Build history of the part. All positions in model axes, mm. A direction names the side the tool comes from. Give positions to 0.01 mm unless a question says otherwise; leave off trailing zeros. Order: outer loops, then holes, each group sorted by start corner. A loop starts at its lowest first (then second) coordinate and runs counter-clockwise, first axis right, second up. Notation, with made-up numbers: (-36, 13.5) - (-23, 13.5) arc R16 ccw to (-23, 41.5) - close; hole circle Ø9 at (19, 47.5). An arc over 180 degrees is marked (long way). Answer in a Markdown table with one row per item.
```python
from build123d import *

# Parameters (mm, degrees)
EXTRUDE_1_DEPTH     = 7
SKETCH_2_R          = 6
CUT_EXTRUDE_1_DEPTH = 5
CUT_EXTRUDE_2_DEPTH = 0.5
FILLET_1_R          = 1
SKETCH_4_R          = 1.5
EXTRUDE_3_DEPTH     = 2.5
SKETCH_5_W          = 1.5
SKETCH_5_H          = 4.3
CUT_EXTRUDE_3_DEPTH = 2.5
SKETCH_6_W          = 3.174285876
SKETCH_6_H          = 3
CUT_EXTRUDE_4_DEPTH = 1


with BuildPart() as part:
    # Эскиз1 → Бобышка-Вытянуть1 (new body)
    with BuildSketch(Plane.XY):
        with BuildLine():
            Line((1.201755047, 83), (6.798244953, 83))
            ThreePointArc((6.798244953, 83), (7.648014096, 82.648014096), (8, 81.798244953))
            Line((8, 81.798244953), (8, 32.201755047))
            ThreePointArc((8, 32.201755047), (7.648014096, 31.351985904), (6.798244953, 31))
            Line((6.798244953, 31), (1.201755047, 31))
            ThreePointArc((1.201755047, 31), (0.351985904, 30.648014096), (0, 29.798244953))
            Line((0, 29.798244953), (0, 1.201755047))
            ThreePointArc((0, 1.201755047), (0.351985904, 0.351985904), (1.201755047, 0))
            Line((1.201755047, 0), (163.798244953, 0))
            ThreePointArc((163.798244953, 0), (164.648014096, 0.351985904), (165, 1.201755047))
            Line((165, 1.201755047), (165, 29.798244953))
            ThreePointArc((165, 29.798244953), (164.648014096, 30.648014096), (163.798244953, 31))
            Line((163.798244953, 31), (158.201755047, 31))
            ThreePointArc((158.201755047, 31), (157.351985904, 31.351985904), (157, 32.201755047))
            Line((157, 32.201755047), (157, 81.798244953))
            ThreePointArc((157, 81.798244953), (157.351985904, 82.648014096), (158.201755047, 83))
            Line((158.201755047, 83), (163.798244953, 83))
            ThreePointArc((163.798244953, 83), (164.648014096, 83.351985904), (165, 84.201755047))
            Line((165, 84.201755047), (165, 111.798244953))
            ThreePointArc((165, 111.798244953), (164.648014096, 112.648014096), (163.798244953, 113))
            Line((163.798244953, 113), (1.201755047, 113))
            ThreePointArc((1.201755047, 113), (0.351985904, 112.648014096), (0, 111.798244953))
            Line((0, 111.798244953), (0, 84.201755047))
            ThreePointArc((0, 84.201755047), (0.351985904, 83.351985904), (1.201755047, 83))
        make_face()
    extrude(amount=EXTRUDE_1_DEPTH)

    # Эскиз2 → Вырез-Вытянуть1 (cut)
    with BuildSketch(Plane(origin=(0, 0, 0), x_dir=(-1, 0, 0), z_dir=(0, 0, -1))):
        with BuildLine():
            Line((-161.798244953, 111), (-3.201755047, 111))
            ThreePointArc((-3.201755047, 111), (-2.351985904, 110.648014096), (-2, 109.798244953))
            Line((-2, 109.798244953), (-2, 86.201755047))
            ThreePointArc((-2, 86.201755047), (-2.351985904, 85.351985904), (-3.201755047, 85))
            Line((-3.201755047, 85), (-8.798244953, 85))
            ThreePointArc((-8.798244953, 85), (-9.648014096, 84.648014096), (-10, 83.798244953))
            Line((-10, 83.798244953), (-10, 30.201755047))
            ThreePointArc((-10, 30.201755047), (-9.648014096, 29.351985904), (-8.798244953, 29))
            Line((-8.798244953, 29), (-3.201755047, 29))
            ThreePointArc((-3.201755047, 29), (-2.351985904, 28.648014096), (-2, 27.798244953))
            Line((-2, 27.798244953), (-2, 3.201755047))
            ThreePointArc((-2, 3.201755047), (-2.351985904, 2.351985904), (-3.201755047, 2))
            Line((-3.201755047, 2), (-161.798244953, 2))
            ThreePointArc((-161.798244953, 2), (-162.648014096, 2.351985904), (-163, 3.201755047))
            Line((-163, 3.201755047), (-163, 27.798244953))
            ThreePointArc((-163, 27.798244953), (-162.648014096, 28.648014096), (-161.798244953, 29))
            Line((-161.798244953, 29), (-156.201755047, 29))
            ThreePointArc((-156.201755047, 29), (-155.351985904, 29.351985904), (-155, 30.201755047))
            Line((-155, 30.201755047), (-155, 70.5))
            Line((-155, 70.5), (-155, 74.8))
            Line((-155, 74.8), (-155, 83.798244953))
            ThreePointArc((-155, 83.798244953), (-155.351985904, 84.648014096), (-156.201755047, 85))
            Line((-156.201755047, 85), (-161.798244953, 85))
            ThreePointArc((-161.798244953, 85), (-162.648014096, 85.351985904), (-163, 86.201755047))
            Line((-163, 86.201755047), (-163, 109.798244953))
            ThreePointArc((-163, 109.798244953), (-162.648014096, 110.648014096), (-161.798244953, 111))
        make_face()
        with Locations((-82.5, 57)):
            Circle(SKETCH_2_R, mode=Mode.SUBTRACT)
    extrude(amount=-CUT_EXTRUDE_1_DEPTH, mode=Mode.SUBTRACT)

    # Эскиз3 → Вырез-Вытянуть2 (cut)
    # profile 1 of 2: a face of its own
    with BuildSketch(Plane(origin=(0, 0, 5), x_dir=(-1, 0, 0), z_dir=(0, 0, -1))):
        with BuildLine():
            Line((-120, 31), (-103, 31))
            ThreePointArc((-103, 31), (-102.292893219, 30.707106781), (-102, 30))
            Line((-102, 30), (-102, 19))
            ThreePointArc((-102, 19), (-102.292893219, 18.292893219), (-103, 18))
            Line((-103, 18), (-120, 18))
            ThreePointArc((-120, 18), (-120.707106781, 18.292893219), (-121, 19))
            Line((-121, 19), (-121, 30))
            ThreePointArc((-121, 30), (-120.707106781, 30.707106781), (-120, 31))
        make_face()
    # profile 2 of 2: a face of its own
    with BuildSketch(Plane(origin=(0, 0, 5), x_dir=(-1, 0, 0), z_dir=(0, 0, -1))):
        with BuildLine():
            Line((-52.1501229, 97.239252875), (-39.1501229, 97.239252875))
            ThreePointArc((-39.1501229, 97.239252875), (-38.443016119, 96.946359657), (-38.1501229, 96.239252875))
            Line((-38.1501229, 96.239252875), (-38.1501229, 83.239252875))
            ThreePointArc((-38.1501229, 83.239252875), (-38.443016119, 82.532146094), (-39.1501229, 82.239252875))
            Line((-39.1501229, 82.239252875), (-52.1501229, 82.239252875))
            ThreePointArc((-52.1501229, 82.239252875), (-52.857229681, 82.532146094), (-53.1501229, 83.239252875))
            Line((-53.1501229, 83.239252875), (-53.1501229, 96.239252875))
            ThreePointArc((-53.1501229, 96.239252875), (-52.857229681, 96.946359657), (-52.1501229, 97.239252875))
        make_face()
        Polygon((-41.403231286, 94.64375803), (-44.490035641, 94.64375803), (-48.784719961, 93.637191392), (-48.784719961, 92.630624755), (-44.490035641, 93.637191392), (-41.403231286, 93.637191392), align=None, mode=Mode.SUBTRACT)
        Polygon((-48.784719961, 91.774831443), (-44.490035641, 92.630624755), (-44.490035641, 91.774831443), (-48.784719961, 90.91903813), align=None, mode=Mode.SUBTRACT)
        Polygon((-48.784719961, 90.055112789), (-44.490035641, 90.910906102), (-44.490035641, 90.055112789), (-48.784719961, 89.067866896), align=None, mode=Mode.SUBTRACT)
        Polygon((-48.784719961, 88.216527408), (-44.490035641, 89.067866896), (-41.403231286, 89.067866896), (-41.403231286, 88.316883581), (-44.341167482, 88.316883581), (-48.784719961, 87.436033812), align=None, mode=Mode.SUBTRACT)
        Polygon((-48.609605566, 93.888102843), (-44.858812452, 94.806018458), (-44.858812452, 95.913847648), (-46.734209009, 95.170019477), (-48.609605566, 95.739760204), align=None, mode=Mode.SUBTRACT)
        Polygon((-48.609605566, 87.006809767), (-44.858812452, 87.715709289), (-44.858812452, 86.328076183), (-46.734209009, 86.674984459), (-48.609605566, 85.770006347), align=None, mode=Mode.SUBTRACT)
    extrude(amount=-CUT_EXTRUDE_2_DEPTH, mode=Mode.SUBTRACT)

    # Скругление1
    fillet_1_edges = [part.edges().sort_by_distance(p)[0] for p in [
        (155, 57, 5),
        (155.351985904, 84.648014096, 5),
        (159, 85, 5),
        (162.648014096, 85.351985904, 5),
        (163, 98, 5),
        (162.648014096, 110.648014096, 5),
        (82.5, 111, 5),
        (2.351985904, 110.648014096, 5),
        (2, 98, 5),
        (2.351985904, 85.351985904, 5),
        (6, 85, 5),
        (9.648014096, 84.648014096, 5),
        (10, 57, 5),
        (9.648014096, 29.351985904, 5),
        (6, 29, 5),
        (2.351985904, 28.648014096, 5),
        (2, 15.5, 5),
        (2.351985904, 2.351985904, 5),
        (82.5, 2, 5),
        (162.648014096, 2.351985904, 5),
        (163, 15.5, 5),
        (162.648014096, 28.648014096, 5),
        (159, 29, 5),
        (155.351985904, 29.351985904, 5),
    ]]
    fillet(fillet_1_edges, radius=FILLET_1_R)

    # Эскиз4 → Бобышка-Вытянуть3 (add)
    # profile 1 of 2: a face of its own
    with BuildSketch(Plane(origin=(0, 0, 0), x_dir=(-1, 0, 0), z_dir=(0, 0, -1))):
        with BuildLine():
            Line((-157, 73), (-163.5, 73))
            ThreePointArc((-163.5, 73), (-164.207106781, 72.707106781), (-164.5, 72))
            Line((-164.5, 72), (-164.5, 41))
            ThreePointArc((-164.5, 41), (-164.207106781, 40.292893219), (-163.5, 40))
            Line((-163.5, 40), (-157, 40))
            Line((-157, 40), (-157, 73))
        make_face()
        with Locations((-161.7, 47)):
            Circle(SKETCH_4_R, mode=Mode.SUBTRACT)
        with Locations((-161.7, 65)):
            Circle(SKETCH_4_R, mode=Mode.SUBTRACT)
    # profile 2 of 2: a face of its own
    with BuildSketch(Plane(origin=(0, 0, 0), x_dir=(-1, 0, 0), z_dir=(0, 0, -1))):
        with BuildLine():
            Line((-1.5, 73), (-8, 73))
            Line((-8, 73), (-8, 40))
            Line((-8, 40), (-1.5, 40))
            ThreePointArc((-1.5, 40), (-0.792893219, 40.292893219), (-0.5, 41))
            Line((-0.5, 41), (-0.5, 72))
            ThreePointArc((-0.5, 72), (-0.792893219, 72.707106781), (-1.5, 73))
        make_face()
        with Locations((-3.3, 47)):
            Circle(SKETCH_4_R, mode=Mode.SUBTRACT)
        with Locations((-3.3, 65)):
            Circle(SKETCH_4_R, mode=Mode.SUBTRACT)
    extrude(amount=-EXTRUDE_3_DEPTH)

    # Эскиз5 → Вырез-Вытянуть3 (cut)
    with BuildSketch(Plane(origin=(0, 0, 0), x_dir=(-1, 0, 0), z_dir=(0, 0, -1))):
        with Locations((-155.75, 72.65)):
            Rectangle(SKETCH_5_W, SKETCH_5_H)
    extrude(amount=-CUT_EXTRUDE_3_DEPTH, mode=Mode.SUBTRACT)

    # Эскиз6 → Вырез-Вытянуть4 (cut)
    with BuildSketch(Plane(origin=(0, 0, 0), x_dir=(-1, 0, 0), z_dir=(0, 0, -1))):
        with Locations((-156.587142938, 81.5)):
            Rectangle(SKETCH_6_W, SKETCH_6_H)
    extrude(amount=-CUT_EXTRUDE_4_DEPTH, mode=Mode.SUBTRACT)


solid = part.part
```
1. Cut at C-C on x = 23.5. Write the cut outline in (y, z).
Check result:
| item | result |
|---|---|
| outline | (0, 0) - (2, 0) - (2, 4) arc R1 cw to (3, 5) - (110, 5) arc R1 cw to (111, 4) - (111, 0) - (113, 0) - (113, 7) - (0, 7) - close |
2. Cut at D-D on y = 25.5. Write the cut outline in (x, z).
Check result:
| item | result |
|---|---|
| outline | (0, 0) - (2, 0) - (2, 4) arc R1 cw to (3, 5) - (102, 5) - (102, 5.5) - (121, 5.5) - (121, 5) - (162, 5) arc R1 cw to (163, 4) - (163, 0) - (165, 0) - (165, 7) - (0, 7) - close |
3. Cut at B-B on y = 99.5. Write the cut outline in (x, z), and give its area (3 significant figures).
Check result:
| item | result |
|---|---|
| outline | (0, 0) - (2, 0) - (2, 4) arc R1 cw to (3, 5) - (162, 5) arc R1 cw to (163, 4) - (163, 0) - (165, 0) - (165, 7) - (0, 7) - close |
| area | 350 mm² |
4. Drop flat-ended pins along their axis: P1, Ø1.5, axis at x = 52, y = 25.5, coming from the -Z side; P2, Ø6, axis at x = 3, y = 54.5, coming from the +Z side; P3, Ø1.2, axis at y = 49.5, z = 1, coming from the +X side. Give the stop position or say it passes through.
Check result:
| item | result |
|---|---|
| P1 | stops at z = 5 |
| P2 | stops at z = 2.5 |
| P3 | stops at x = 164.5 |
5. Cut at A-A on x = 82.5. Write the cut outline in (y, z), and give its area (3 significant figures).
Check result:
| item | result |
|---|---|
| outline | (0, 0) - (2, 0) - (2, 4) arc R1 cw to (3, 5) - (51, 5) - (51, 0) - (63, 0) - (63, 5) - (110, 5) arc R1 cw to (111, 4) - (111, 0) - (113, 0) - (113, 7) - (0, 7) - close |
| area | 306 mm² |
6. Which spindle directions (+Z, -Z, +X, -X, +Y, -Y) get a long thin tool onto all of the face, cutting with end or side? Do faces 4 (the face through (4, 57, 2.5)), 5 (the face through (161, 57, 2.5)), 6 (the face through (2, 98, 2)). Say none if no direction does.
Check result:
| item | result |
|---|---|
| face 4 | +Z, -X |
| face 5 | +Z, +X |
| face 6 | -Z |
7. Probe line 1 (X direction, y = 65, z = 0.9); line 2 (Y direction, x = 8.5, z = 2); line 3 (X direction, y = 53, z = 2.75). List the from-to ranges inside material, lowest first.
Check result:
| item | result |
|---|---|
| line 1 | x = 0.5 to 1.8, 4.8 to 10, 155 to 160.2, 163.2 to 164.5 |
| line 2 | y = 0 to 2, 29 to 85, 111 to 113 |
| line 3 | x = 8 to 10, 78.03 to 86.97, 155 to 157 |
8. Two-plate mould, pull along Y, no slides. Class faces 1 (the face through (0, 16, 3)), 2 (the face through (157, 57, 4)), 3 (the face through (81, 0, 3)): +Y half, -Y half, draft (parallel to the pull), parting line (faces both ways), or undercut.
Check result:
| item | result |
|---|---|
| face 1 | draft |
| face 2 | undercut |
| face 3 | -Y half |
